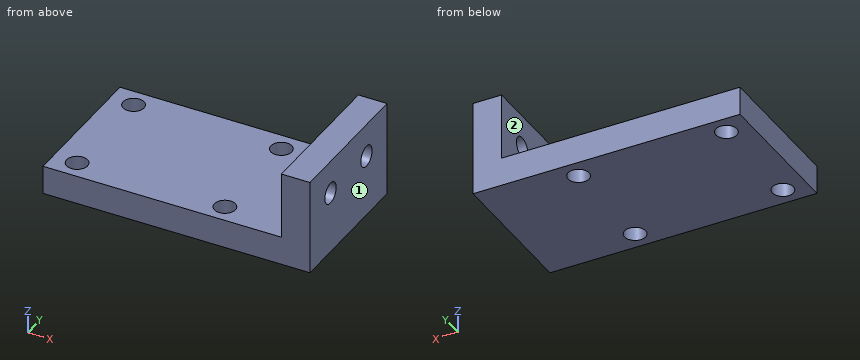
Autodesk Inventor part; units mm, degrees
ref_plane "YZ Plane" through (0, 0, 0) normal (1, 0, 0) x (0, 1, 0)
ref_plane "XZ Plane" through (0, 0, 0) normal (0, 1, 0) x (-1, 0, 0)
ref_plane "XY Plane" through (0, 0, 0) normal (0, 0, 1) x (1, 0, 0)
sketch "スケッチ1" plane through (0, 0, 0) normal (0, 0, 1) x (1, 0, 0)
  line L0 (-14, -7.5) -> (14, -7.5)
  line L1 (14, -7.5) -> (14, 7.5)
  line L2 (14, 7.5) -> (-14, 7.5)
  line L3 (-14, 7.5) -> (-14, -7.5)
  line L4 (-14, -7.5) -> (14, 7.5) construction
  line L5 (14, -7.5) -> (-14, 7.5) construction
  point P0 (0, 0)
  dimension "d0" = 28
  dimension "d1" = 15
extrude "押し出し1" add sketch "スケッチ1" along normal mid plane 3
sketch "スケッチ2" plane through (0, 0, 1.5) normal (0, 0, 1) x (1, 0, 0)
  line L0 (14, -7.5) -> (14, 7.5)
  line L1 (-14, -7.5) -> (14, -7.5)
  line L2 (14, 7.5) -> (11, 7.5)
  line L3 (11, 7.5) -> (11, -7.5)
  line L4 (11, -7.5) -> (14, -7.5)
  line L5 (14, -7.5) -> (14, 7.5)
  point P0 (0, 0)
  dimension "d4" = 3
extrude "押し出し2" add sketch "スケッチ2" along normal blind 7
sketch "スケッチ3" plane through (0, 0, 1.5) normal (0, 0, 1) x (1, 0, 0)
  line L0 (-14, 7.5) -> (-14, -7.5)
  line L1 (0, 0) -> (-2.791, 0)
  point P0 (-11.5, 5.5)
  point P1 (4, 5.5)
  point P2 (-11.5, -5.5)
  point P3 (4, -5.5)
  dimension "d7" = 15.5
  dimension "d8" = 2.5
  dimension "d9" = 5.5
  dimension "d10" = 5.5
hole "穴1" at (-11.5, 5.5, 1.5) at (4, 5.5, 1.5) at (-11.5, -5.5, 1.5) at (4, -5.5, 1.5) direction (0, 0, -1) diameter 2.2 end through all
sketch "スケッチ4" plane through (11, -7.5, 1.5) normal (-1, 0, 0) x (0, 0, 1)
  line L0 (0, 15) -> (7, 15)
  line L1 (7, 15) -> (7, 0)
  line L2 (0, 0) -> (7, 0)
  point P0 (-1.5, 7.5)
  point P1 (3.5, 11)
  point P2 (3.5, 4)
  dimension "d18" = 4
  dimension "d19" = 3.5
  dimension "d20" = 3.5
  dimension "d21" = 4
hole "穴2" at (11, 3.5, 5) at (11, -3.5, 5) direction (1, 0, 0) diameter 2.2 end through all
properties part number "sponge_holder"
Geometry check sheet. Reference: the model listing, model coordinates, mm. Face numbers are marked on the shaded views. A direction names the side the tool comes from. Give positions to 0.01 mm unless a question says otherwise; leave off trailing zeros. Loops run counter-clockwise (first coordinate to the right, second up) from the corner with the lowest first, then second, coordinate; pieces in that order, holes last. Notation, with made-up numbers: M 57,-8.75 L 70,-8.75 A31 cw 70,16.25 Z; hole C 16,75.25 d11. An arc over 180 degrees is marked long. Write item = value, one per line.
(1) Sectioned sample at C-C, the plane x = 4. Record the cut outline in (y, z).
Answer below:
outline = M -7.5,-1.5 L -6.6,-1.5 L -6.6,1.5 L -7.5,1.5 Z; M -4.4,-1.5 L 4.4,-1.5 L 4.4,1.5 L -4.4,1.5 Z; M 6.6,-1.5 L 7.5,-1.5 L 7.5,1.5 L 6.6,1.5 Z
(2) Gauge pin test, flat ends, axial feed: pin 1 Ø2 at (x, y) = (9.5, 3.5) entering from +Z; pin 2 Ø2 at (y, z) = (4.5, 6) entering from -X; pin 3 Ø1.8 at (x, y) = (-11.5, 5.5) entering from +Z. Record the tip position at first contact, or that the pin passes through.
Answer below:
pin_1 = 1.5
pin_2 = 11
pin_3 = through
(3) Sectioned sample at D-D, the plane z = 0.25. Record the cut outline in (x, y).
Answer below:
outline = M -14,-7.5 L 14,-7.5 L 14,7.5 L -14,7.5 Z; hole C -11.5,-5.5 d2.2; hole C -11.5,5.5 d2.2; hole C 4,-5.5 d2.2; hole C 4,5.5 d2.2
(4) Sectioned sample at B-B, the plane y = -3.5. Record the cut outline in (x, z), plus the area to 3 significant figures.
Answer below:
outline = M -14,-1.5 L 14,-1.5 L 14,3.9 L 11,3.9 L 11,1.5 L -14,1.5 Z; M 11,6.1 L 14,6.1 L 14,8.5 L 11,8.5 Z
area = 98.4 mm2
(5) Material ranges on line 1 (Y direction, x = -11.5, z = 0); line 2 (X direction, y = 5.5, z = -0.4); line 3 (Z direction, x = 13.05, y = -3.5), recorded low to high. Write a range as [from, to].
Answer below:
line_1 = [-7.5, -6.6], [-4.4, 4.4], [6.6, 7.5]
line_2 = [-14, -12.6], [-10.4, 2.9], [5.1, 14]
line_3 = [-1.5, 3.9], [6.1, 8.5]
(6) Tool access check on the marked faces 1 and 2. Record the directions out of +Z, -Z, +X, -X, +Y, -Y that give a thin tool (end or side, any length) a straight path to the whole face; none if there is none.
Answer below:
face_1 = +Z, -Z, +X, +Y, -Y
face_2 = +Z, -X, +Y, -Y
(7) Sectioned sample at A-A, the plane z = 5. Record the cut outline in (x, y).
Answer below:
outline = M 11,-7.5 L 14,-7.5 L 14,-4.6 L 11,-4.6 Z; M 11,-2.4 L 14,-2.4 L 14,2.4 L 11,2.4 Z; M 11,4.6 L 14,4.6 L 14,7.5 L 11,7.5 Z
